```python
from build123d import *

# Parameters (mm, degrees)
SKETCH1_W           = 340
SKETCH1_H           = 195
BOSS_EXTRUDE1_DEPTH = 2
SKETCH2_R           = 2.5
CUT_EXTRUDE1_DEPTH  = 3
LPATTERN1_COUNT     = 2
LPATTERN1_PITCH     = 10
LPATTERN1_COL_COUNT = 3
LPATTERN1_COL_PITCH = 10
CUT_EXTRUDE2_DEPTH  = 3
SKETCH4_W           = 55
SKETCH4_H           = 55
CUT_EXTRUDE3_DEPTH  = 3
FILLET1_R           = 10
FILLET2_R           = 10


with BuildPart() as part:
    # Sketch1 → Boss-Extrude1 (new body)
    with BuildSketch(Plane.XY):
        with Locations((-439.9, -389.5)):
            Rectangle(SKETCH1_W, SKETCH1_H)
    extrude(amount=BOSS_EXTRUDE1_DEPTH)

    # Sketch2 → Cut-Extrude1 (cut, through all)
    with BuildSketch(Plane.XY.offset(2)):
        with Locations((-449.8, -362)):
            Circle(SKETCH2_R)
        with Locations((-449.8, -462)):
            Circle(SKETCH2_R)
        with Locations((-549.8, -462)):
            Circle(SKETCH2_R)
        with Locations((-549.8, -362)):
            Circle(SKETCH2_R)
    cut_extrude1 = extrude(amount=-CUT_EXTRUDE1_DEPTH, mode=Mode.SUBTRACT)

    # LPattern1: Cut-Extrude1 ×2
    with Locations(*[(0, -i * LPATTERN1_PITCH, 0) for i in range(1, LPATTERN1_COUNT)]):
        add(cut_extrude1, mode=Mode.SUBTRACT)

    # LPattern1 col: Cut-Extrude1 ×3
    with Locations(*[(0, i * LPATTERN1_COL_PITCH, 0) for i in range(1, LPATTERN1_COL_COUNT)]):
        add(cut_extrude1, mode=Mode.SUBTRACT)

    # Sketch3 → Cut-Extrude2 (cut, through all)
    with BuildSketch(Plane.XY.offset(2)):
        Polygon((-307.57766953, -457), (-357.4, -407.17766953), (-407.22233047, -457), align=None)
        Polygon((-289.9, -439.32233047), (-339.72233047, -389.5), (-289.9, -339.67766953), align=None)
        Polygon((-375.07766953, -389.5), (-424.9, -439.32233047), (-424.9, -339.67766953), align=None)
        Polygon((-357.4, -371.82233047), (-307.57766953, -322), (-407.22233047, -322), align=None)
    extrude(amount=-CUT_EXTRUDE2_DEPTH, mode=Mode.SUBTRACT)

    # Sketch4 → Cut-Extrude3 (cut, through all)
    with BuildSketch(Plane.XY.offset(2)):
        with Locations((-499.8, -429.5)):
            Rectangle(SKETCH4_W, SKETCH4_H)
        with Locations((-499.8, -349.5)):
            Rectangle(SKETCH4_W, SKETCH4_H)
    extrude(amount=-CUT_EXTRUDE3_DEPTH, mode=Mode.SUBTRACT)

    # Fillet1
    fillet1_edges = [part.edges().sort_by_distance(p)[0] for p in [
        (-289.9, -339.67766953, 1),
        (-289.9, -439.32233047, 1),
        (-339.72233047, -389.5, 1),
        (-424.9, -339.67766953, 1),
        (-375.07766953, -389.5, 1),
        (-424.9, -439.32233047, 1),
        (-357.4, -371.82233047, 1),
        (-407.22233047, -322, 1),
        (-307.57766953, -322, 1),
        (-307.57766953, -457, 1),
        (-407.22233047, -457, 1),
        (-357.4, -407.17766953, 1),
        (-472.3, -402, 1),
        (-472.3, -457, 1),
        (-527.3, -457, 1),
        (-527.3, -402, 1),
        (-472.3, -322, 1),
        (-472.3, -377, 1),
        (-527.3, -377, 1),
        (-527.3, -322, 1),
    ]]
    fillet(fillet1_edges, radius=FILLET1_R)

    # Fillet2
    fillet2_edges = [part.edges().sort_by_distance(p)[0] for p in [
        (-269.9, -487, 1),
        (-609.9, -487, 1),
        (-609.9, -292, 1),
        (-269.9, -292, 1),
    ]]
    fillet(fillet2_edges, radius=FILLET2_R)


solid = part.part
```
Check sheet for the modelled part. Datum: model origin and axes. Units: mm. A direction names the side the tool comes from. Round coordinates to 2 decimals unless told otherwise and drop trailing zeros. Order: outer loops, then holes, each group sorted by start corner. A loop starts at its lowest first (then second) coordinate and runs counter-clockwise, first axis right, second up.
1) Section check C-C (x = -417). Record the boundary of the cut face in (y, z).
2) Mould release check, pull along Y, two halves, no side actions. Record for faces 3 (the cylindrical face through (-392.255, -450.979, 0.986)), 4 (the cylindrical face through (-322.419, -328.326, 0.986)), 5 (the flat face through (-442, -388, 0)), 6 (the cylindrical face through (-272.91, -484.15, 1.01)): +Y half, -Y half, draft (parallel to the pull), parting line (faces both ways), or undercut.
3) Scan lines: line 1 (Y direction, x = -504.5, z = 1.95); line 2 (X direction, y = -462, z = 1); line 3 (X direction, y = -323, z = 1.75). Record each from-to range of solid material in increasing order.
4) Section check B-B (y = -390). Record the boundary of the cut face in (x, z), and give its area (3 significant figures).
5) Go/stop test with a flat-tipped pin: pin 1 Ø8 at (x, y) = (-549.8, -372) entering from -Z. Record where the tip stops, or that it passes through.
6) Section check D-D (z = 0.3). Give the number of separate pieces and of enclosed holes in the cut face, and give its area (3 significant figures).
7) Section check A-A (x = -499). Record the boundary of the cut face in (y, z), and give its area (3 significant figures).
8) Tool access check on faces 1 (the cylindrical face through (-524.29, -454.15, 0.99)), 2 (the cylindrical face through (-607.05, -295.01, 1.01)). Record the directions out of +Z, -Z, +X, -X, +Y, -Y that give a thin tool (end or side, any length) a straight path to the whole face; none if there is none.
Result:
1. outline: (-487, 0) - (-424.96, 0) - (-424.96, 2) - (-487, 2) - close; (-354.04, 0) - (-292, 0) - (-292, 2) - (-354.04, 2) - close
2. face 3: undercut
2. face 4: undercut
2. face 5: draft
2. face 6: -Y half
3. line 1: y = -487 to -457, -402 to -377, -322 to -292
3. line 2: x = -609.9 to -552.3, -547.3 to -452.3, -447.3 to -269.9
3. line 3: x = -609.9 to -521.66, -477.94 to -387.44, -327.36 to -269.9
4. outline: (-609.9, 0) - (-424.9, 0) - (-424.9, 2) - (-609.9, 2) - close; (-379.23, 0) - (-335.57, 0) - (-335.57, 2) - (-379.23, 2) - close; (-289.9, 0) - (-269.9, 0) - (-269.9, 2) - (-289.9, 2) - close
4. area: 497 mm2
5. pin 1: stops at z = 0
6. separate pieces: 1
6. enclosed holes: 22
6. area: 51,200 mm2
7. outline: (-487, 0) - (-457, 0) - (-457, 2) - (-487, 2) - close; (-402, 0) - (-377, 0) - (-377, 2) - (-402, 2) - close; (-322, 0) - (-292, 0) - (-292, 2) - (-322, 2) - close
7. area: 170 mm2
8. face 1: +Z, -Z
8. face 2: +Z, -Z, -X, +Y
